Input: dimensioned drawing with shaded views. Units: mm. Origin: part minimum x, y, z. A direction names the side the tool comes from. Coordinates: 2 decimals unless noted, no trailing zeros. Loops run counter-clockwise (first coordinate to the right, second up) from the corner with the lowest first, then second, coordinate; pieces in that order, holes last. Notation, with made-up numbers: (26, 2.25) - (35, 2.25) arc R15 cw to (35, 6.25) - close; hole circle Ø3 at (-14.5, -8). An arc over 180 degrees is marked (long way). Use one line per item in the form item = value. Start each with the question number.
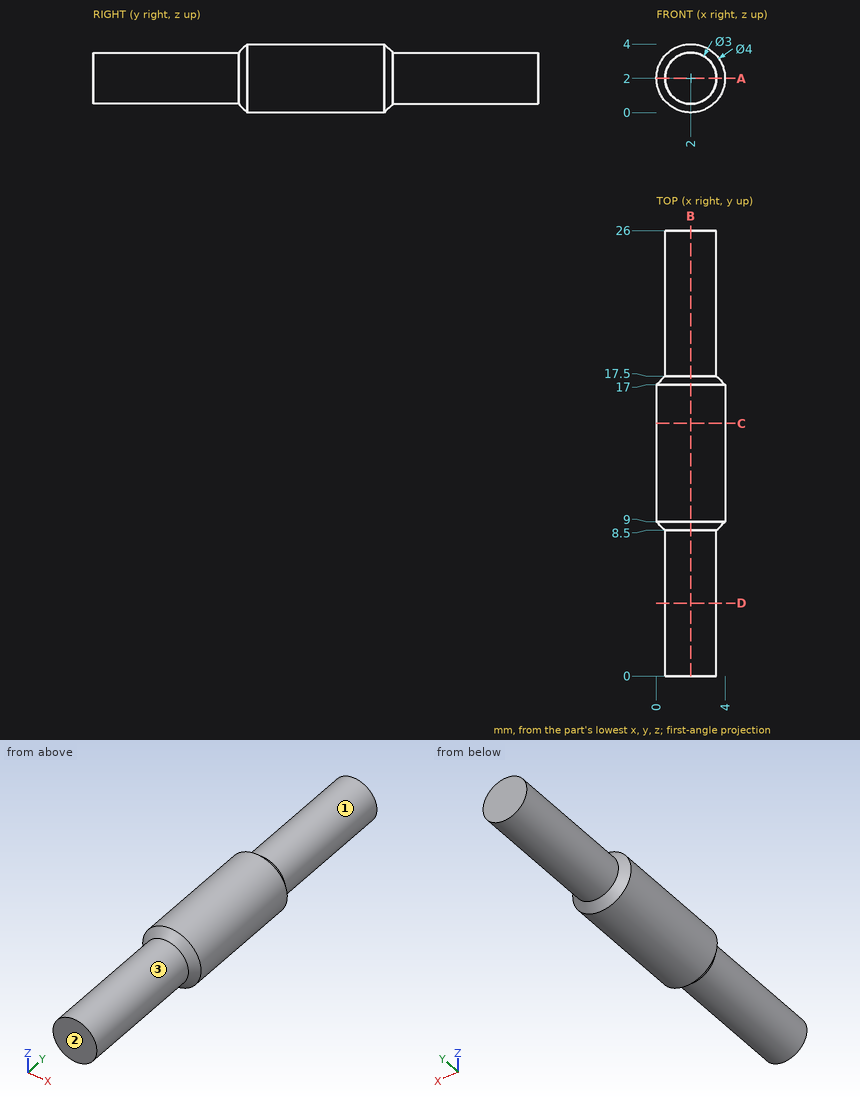
(1) Access query for the marked faces 1, 2 and 3. Directions: +Z, -Z, +X, -X, +Y, -Y. A direction counts if a zero-diameter tool reaches every point of the face in a straight line with its end or side. Return the directions, or none.
(2) Cut plane B-B, the plane x = 2. Output: boundary loops of the cut face in (y, z).
(3) Material intervals for line 1 (X direction, y = 16.75, z = 2.15); line 2 (X direction, y = 4.5, z = 0.9); line 3 (Z direction, x = 1.6, y = 12), sorted ascending.
(4) Cut plane C-C, the plane y = 14.75. Output: boundary loops of the cut face in (x, z), plus the area to 3 significant figures.
(5) Cut plane D-D, the plane y = 4.25. Output: boundary loops of the cut face in (x, z).
(6) Contact query for a flat-ended pin moving along its axis: pin 1 (1 mm diameter, centred on y = 16.5, z = 1, fed in from -X). Output: stop coordinate, or through.
(7) Cut plane A-A, the plane z = 2. Output: boundary loops of the cut face in (x, y), plus the area to 3 significant figures.
Recorded:
q1.face_1 = +Y
q1.face_2 = +Z, -Z, +X, -X, -Y
q1.face_3 = -Y
q2.outline = (0, 0.5) - (8.5, 0.5) - (9, 0) - (17, 0) - (17.5, 0.5) - (26, 0.5) - (26, 3.5) - (17.5, 3.5) - (17, 4) - (9, 4) - (8.5, 3.5) - (0, 3.5) - close
q3.line_1 = 0.01 to 3.99
q3.line_2 = 0.98 to 3.02
q3.line_3 = 0.04 to 3.96
q4.outline = circle Ø4 at (2, 2)
q4.area = 12.6 mm²
q5.outline = circle Ø3 at (2, 2)
q6.pin_1 = 0.06
q7.outline = (0, 9) - (0.5, 8.5) - (0.5, 0) - (3.5, 0) - (3.5, 8.5) - (4, 9) - (4, 17) - (3.5, 17.5) - (3.5, 26) - (0.5, 26) - (0.5, 17.5) - (0, 17) - close
q7.area = 86.5 mm²
